Model file for the job. Use its own axes, mm. Face numbers are marked on the shaded views. A direction names the side the tool comes from. Coordinates: 2 decimals unless noted, no trailing zeros. Order: outer loops, then holes, each group sorted by start corner. A loop starts at its lowest first (then second) coordinate and runs counter-clockwise, first axis right, second up. Notation, with made-up numbers: (79.5, 31) -> (125.5, 31) arc R29 ccw to (125.5, 58) -> close; hole circle Ø7 at (76, 55). An arc over 180 degrees is marked (long way). Use CSV: the item, a comma, the result in double quotes. Start each with the question number.
(1) Cut at A-A on y = 39.75. Write the cut outline in (x, z).
(2) Pull direction X, two halves, no side cores. Call the marked faces 1, 2, 3 and 4: pulls with the +X half, pulls with the -X half, needs draft (parallel to the pull), parting line crosses it, or undercut.
(3) Cut at C-C on z = -2.5. Write the cut outline in (x, y).
(4) Tool access for the marked faces 5 and 6: list every direction of +Z, -Z, +X, -X, +Y, -Y with a clear straight run to the whole face (end or side of a thin tool).
(5) Pin check, flat tips, straight feed: pin 1 Ø7 at (x, y) = (6.5, 39.75) entering from +Z; pin 2 Ø3 at (x, z) = (-3.5, -2) entering from -Y. Stop position of each tip, or through.
(6) Cut at B-B on x = 0. Write the cut outline in (y, z).
(7) Probe L1, parallel to X at y = 40, z = -1.7; L2, parallel to X at y = 38, z = -3.3; L3, parallel to X at y = 45, z = -3.8. List the from-to ranges inside material, lowest first.
```python
from build123d import *

# Parameters (mm, degrees)
F0_R     = 4.75
F0_R_2   = 4
F0_R_3   = 2.35
F1_DEPTH = 6
F2_DEPTH = 4
F3_R     = 5
F4_R     = 1


with BuildPart() as f1:
    # F0 (on Top) → F1 (new body)
    with BuildSketch(Plane.XY):
        with BuildLine():
            Line((12.5, 49.75), (-12.5, 49.75))
            Line((-12.5, 49.75), (-12.5, 29.75))
            Line((-12.5, 29.75), (-8.683703, -1.075085))
            ThreePointArc((-8.683703, -1.075085), (0, -8.75), (8.683703, -1.075085))
            Line((8.683703, -1.075085), (12.5, 29.75))
            Line((12.5, 29.75), (12.5, 49.75))
        make_face()
        Circle(F0_R, mode=Mode.SUBTRACT)
        with Locations((-6.5, 39.75)):
            Circle(F0_R_2, mode=Mode.SUBTRACT)
        with Locations((6.5, 39.75)):
            Circle(F0_R_2, mode=Mode.SUBTRACT)
        with Locations((-6.5, 39.75)):
            Circle(F0_R_2)
        with Locations((-6.5, 39.75)):
            Circle(F0_R_3, mode=Mode.SUBTRACT)
        with Locations((6.5, 39.75)):
            Circle(F0_R_2)
        with Locations((6.5, 39.75)):
            Circle(F0_R_3, mode=Mode.SUBTRACT)
    extrude(amount=-F1_DEPTH)

    # F0 (on Top) → F2 (cut)
    with BuildSketch(Plane.XY):
        with Locations((-6.5, 39.75)):
            Circle(F0_R_2)
        with Locations((-6.5, 39.75)):
            Circle(F0_R_3, mode=Mode.SUBTRACT)
        with Locations((6.5, 39.75)):
            Circle(F0_R_2)
        with Locations((6.5, 39.75)):
            Circle(F0_R_3, mode=Mode.SUBTRACT)
    extrude(amount=-F2_DEPTH, mode=Mode.SUBTRACT)

    # F3
    f3_edges = [f1.edges().sort_by_distance(p)[0] for p in [
        (-12.5, 49.75, -3),
        (12.5, 49.75, -3),
        (-12.5, 29.75, -3),
        (12.5, 29.75, -3),
    ]]
    fillet(f3_edges, radius=F3_R)

    # F4
    f4_edges = [f1.edges().sort_by_distance(p)[0] for p in [
        (-10.572909, 14.184458, 0),
    ]]
    fillet(f4_edges, radius=F4_R)


solid = f1.part
```
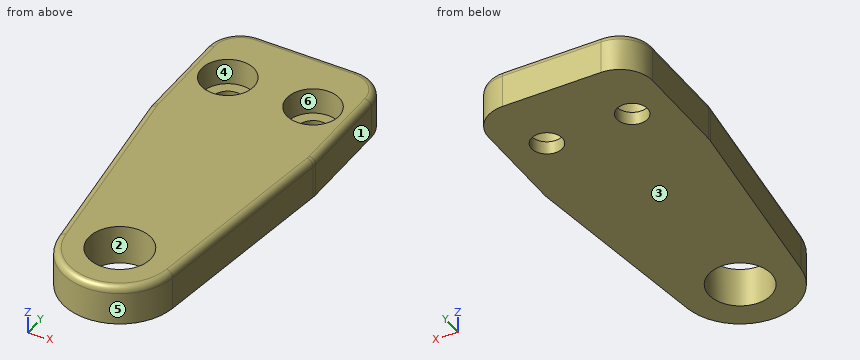
Outcome:
1,outline,"(-12.5, -6) -> (-8.85, -6) -> (-8.85, -4) -> (-10.5, -4) -> (-10.5, 0) -> (-11.5, 0) arc R1 ccw to (-12.5, -1) -> close; (-4.15, -6) -> (4.15, -6) -> (4.15, -4) -> (2.5, -4) -> (2.5, 0) -> (-2.5, 0) -> (-2.5, -4) -> (-4.15, -4) -> close; (8.85, -6) -> (12.5, -6) -> (12.5, -1) arc R1 ccw to (11.5, 0) -> (10.5, 0) -> (10.5, -4) -> (8.85, -4) -> close"
2,face 1,"pulls with the +X half"
2,face 2,"undercut"
2,face 3,"needs draft"
2,face 4,"undercut"
3,outline,"(-12.5, 30.06) arc R5 ccw to (-12.46, 29.44) -> (-8.68, -1.08) arc R8.75 ccw to (8.68, -1.08) -> (12.46, 29.44) arc R5 ccw to (12.5, 30.06) -> (12.5, 44.75) arc R5 ccw to (7.5, 49.75) -> (-7.5, 49.75) arc R5 ccw to (-12.5, 44.75) -> close; hole circle Ø8 at (-6.5, 39.75); hole circle Ø9.5 at (0, 0); hole circle Ø8 at (6.5, 39.75)"
4,face 5,"+Z, -Z, -Y"
4,face 6,"+Z"
5,pin 1,"z = -4"
5,pin 2,"y = -8.52"
6,outline,"(-8.75, -6) -> (-4.75, -6) -> (-4.75, 0) -> (-7.75, 0) arc R1 ccw to (-8.75, -1) -> close; (4.75, -6) -> (49.75, -6) -> (49.75, -1) arc R1 ccw to (48.75, 0) -> (4.75, 0) -> close"
7,L1,"-12.5 to -10.49, -2.51 to 2.51, 10.49 to 12.5"
7,L2,"-12.5 to -10.1, -2.9 to 2.9, 10.1 to 12.5"
7,L3,"-12.49 to 12.49"
